```python
from build123d import *

# Parameters (mm, degrees)
F1_DEPTH      = 25.4
F3_DEPTH      = 6.35
F3_DEPTH_BACK = 12.7
F4_DEPTH      = 6.35
F4_DEPTH_BACK = 25.4
F7_DEPTH      = 12.7
F8_R          = 3.175
F9_DEPTH      = 69.851


with BuildPart() as f1:
    # F0 (on Front) → F1 (new body, symmetric)
    with BuildSketch(Plane.XZ):
        Polygon((25.4, 0), (76.2, 0), (76.2, 50.8), (38.1, 57.15), (0, 57.15), (0, 25.4), align=None)
    extrude(amount=F1_DEPTH, both=True)


with BuildPart() as f3:
    # F2 (on Front) → F3 (new body, two sides)
    with BuildSketch(Plane.XZ) as f3_sk:
        Polygon((76.2, 50.8), (76.2, 31.75), (101.6, 31.75), (101.6, 69.85), (63.5, 69.85), (63.5, 52.9166666667), align=None)
    extrude(amount=F3_DEPTH)
    extrude(f3_sk.sketch, amount=-F3_DEPTH_BACK)


with BuildPart() as f4:
    # F2 (on Front) → F4 (new body, two sides)
    with BuildSketch(Plane.XZ) as f4_sk:
        Polygon((76.2, 31.75), (76.2, 0), (114.3, 0), (114.3, 25.4), (101.6, 31.75), align=None)
    extrude(amount=F4_DEPTH)
    extrude(f4_sk.sketch, amount=-F4_DEPTH_BACK)


with BuildPart() as f3_1:
    add(f3.part)

    # F5: union F4, F1
    add(f4.part)
    add(f1.part)

    # F6 (on face) → F7 (join, through all)
    with BuildSketch(Plane(origin=(0, 25.4, 0), x_dir=(-1, 0, 0), z_dir=(0, 1, 0))):
        Polygon((-76.2, 31.75), (-76.2, 50.8), (-101.6, 31.75), align=None)
    extrude(amount=-F7_DEPTH)

    # F8 (on face) → F9 (cut, through all)
    with BuildSketch(Plane.XY.offset(69.85)):
        with Locations((92.075, 3.175)):
            Circle(F8_R)
        with Locations((73.025, 3.175)):
            Circle(F8_R)
    extrude(amount=-F9_DEPTH, mode=Mode.SUBTRACT)


solid = f3_1.part
```
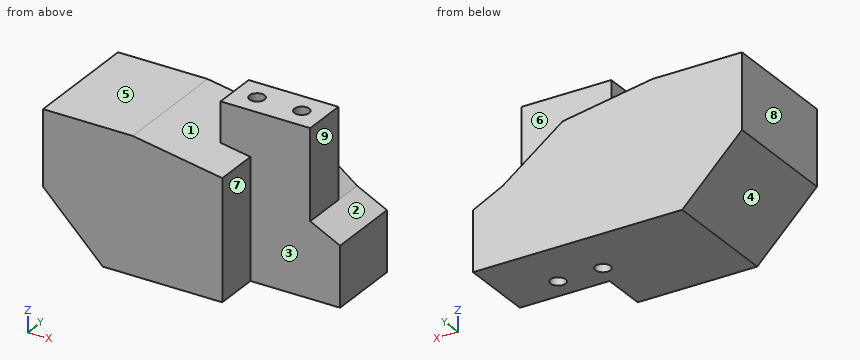
Verification items for the finished model (mm, model axes). Face numbers are marked on the shaded views. A direction names the side the tool comes from. Coordinates: 2 decimals unless noted, no trailing zeros. Loops run counter-clockwise (first coordinate to the right, second up) from the corner with the lowest first, then second, coordinate; pieces in that order, holes last. Notation, with made-up numbers: (-19.75, 64) -> (1.25, 64) arc R5 cw to (1.25, 72) -> close; hole circle Ø7 at (27, 77). An arc over 180 degrees is marked (long way). Answer in a Markdown table with one row per item. Add a question column.
1. Draft check along X on the marked faces 1, 2, 3 and 4. Enter one of: +X half, -X half, draft (parallel to the pull), parting line (faces both ways), or undercut.
2. Section check A-A, the plane y = 10. Enter the section's corners in (x, z).
3. Section check B-B, the plane x = 94. Enter the section's corners in (y, z).
4. Section check D-D, the plane x = 32. Enter the section's corners in (y, z), then the cut area to 3 significant figures.
5. Material ranges on probe 1 along X at (y, z) = (3, 47); probe 2 along X at (y, z) = (1.5, 60.5); probe 3 along Y at (x, z) = (73, 26), recorded low to high. Write a range as [from, to].
6. Depth check by flat-ended pin: P1, Ø9.5, axis at y = -15, z = 37, coming from the +X side; P2, Ø1, axis at x = 33.5, y = 18, coming from the +Z side; P3, Ø5, axis at y = 1.5, z = 65, coming from the -X side; P4, Ø5.5, axis at x = 73.025, y = 3.175, coming from the +Z side. Enter the tip coordinate at first touch or a pass-through.
7. Section check C-C, the plane z = 7. Enter the section's corners in (x, y) (3 decimals), then the cut area to 3 significant figures.
8. Access from +Z, -Z, +X, -X, +Y, -Y to the whole of each face (thin tool, end or side, straight path). Record for the marked faces 5, 6, 7, 8 and 9.
Derived:
| question | item | result |
|---|---|---|
| 1 | face 1 | undercut |
| 1 | face 2 | +X half |
| 1 | face 3 | draft |
| 1 | face 4 | -X half |
| 2 | outline | (0, 25.4) -> (25.4, 0) -> (114.3, 0) -> (114.3, 25.4) -> (101.6, 31.75) -> (101.6, 69.85) -> (63.5, 69.85) -> (63.5, 52.92) -> (38.1, 57.15) -> (0, 57.15) -> close |
| 3 | outline | (-6.35, 0) -> (0.65, 0) -> (0.65, 69.85) -> (-6.35, 69.85) -> close; (5.7, 0) -> (25.4, 0) -> (25.4, 37.45) -> (12.7, 37.45) -> (12.7, 69.85) -> (5.7, 69.85) -> close |
| 4 | outline | (-25.4, 0) -> (25.4, 0) -> (25.4, 57.15) -> (-25.4, 57.15) -> close |
| 4 | area | 2,900 mm² |
| 5 | probe 1 | x = [0, 69.85], [76.2, 88.9], [95.25, 101.6] |
| 5 | probe 2 | x = [63.5, 70.33], [75.72, 89.38], [94.77, 101.6] |
| 5 | probe 3 | y = [-25.4, 0], [6.35, 25.4] |
| 6 | P1 | stops at x = 76.2 |
| 6 | P2 | stops at z = 57.15 |
| 6 | P3 | stops at x = 63.5 |
| 6 | P4 | passes through |
| 7 | outline | (18.4, -25.4) -> (76.2, -25.4) -> (76.2, -6.35) -> (114.3, -6.35) -> (114.3, 25.4) -> (18.4, 25.4) -> close; hole circle Ø6.35 at (73.025, 3.175); hole circle Ø6.35 at (92.075, 3.175) |
| 7 | area | 4,080 mm² |
| 8 | face 5 | +Z, -X, +Y, -Y |
| 8 | face 6 | +Z, +X, +Y |
| 8 | face 7 | +Z, -Z, +X, -Y |
| 8 | face 8 | +Z, -Z, -X, +Y, -Y |
| 8 | face 9 | +Z, +X, +Y, -Y |
